Print and shaded views of the part. All mm, measured from the part's lowest x, y and z. A direction names the side the tool comes from. Round coordinates to 2 decimals unless told otherwise and drop trailing zeros. Loops run counter-clockwise (first coordinate to the right, second up) from the corner with the lowest first, then second, coordinate; pieces in that order, holes last. Notation, with made-up numbers: (25, 78) -> (58, 78) arc R26 ccw to (58, 96) -> close; hole circle Ø8 at (-14, 58.25). An arc over 180 degrees is marked (long way). Answer as CSV lines item,"result".
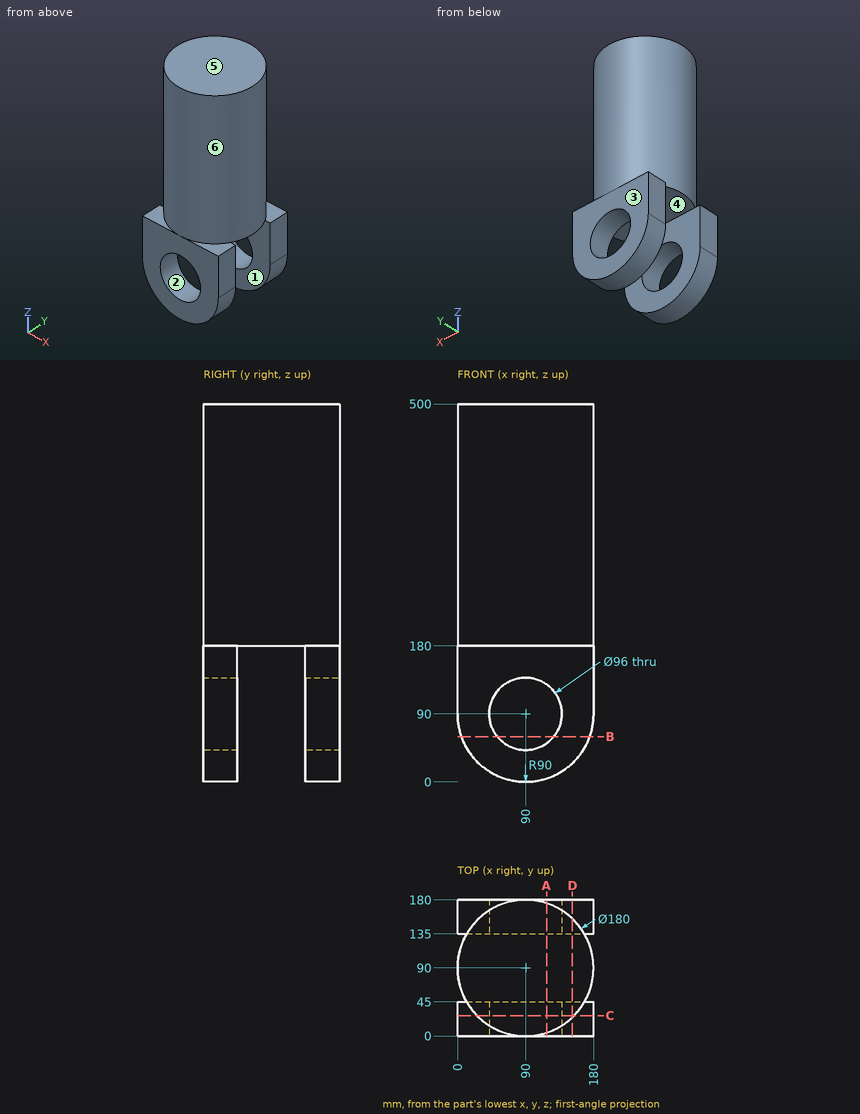
Q1. Drop flat-ended pins along their axis: pin 1 Ø8 at (x, y) = (55.5, 110.5) entering from -Z; pin 2 Ø12 at (x, z) = (27, 105.5) entering from -Y; pin 3 Ø1.5 at (x, z) = (84, 189.5) entering from +Y; pin 4 Ø1 at (x, z) = (69, 349.5) entering from +Y. Give the stop position or say it passes through.
Results:
pin 1,"z = 180"
pin 2,"y = 0"
pin 3,"y = 179.85"
pin 4,"y = 177.63"
Q2. Slice it at A-A, the plane x = 118. Give the cut face in (y, z), and give its area (3 significant figures).
Results:
outline,"(0, 4.47) -> (45, 4.47) -> (45, 51.01) -> (0, 51.01) -> close; (0, 128.99) -> (45, 128.99) -> (45, 180) -> (135, 180) -> (135, 128.99) -> (180, 128.99) -> (180, 180) -> (175.53, 180) -> (175.53, 500) -> (4.47, 500) -> (4.47, 180) -> (0, 180) -> close; (135, 4.47) -> (180, 4.47) -> (180, 51.01) -> (135, 51.01) -> close"
area,"63,500 mm2"
Q3. Slice it at C-C, the plane y = 27. Give the cut face in (x, z), and give its area (3 significant figures).
Results:
outline,"(0, 90) arc R90 ccw to (180, 90) -> (180, 180) -> (154.27, 180) -> (154.27, 500) -> (25.73, 500) -> (25.73, 180) -> (0, 180) -> close; hole circle Ø96 at (90, 90)"
area,"62,800 mm2"
Q4. Probe L1, parallel to Z at x = 90, y = 145; L2, parallel to X at y = 9, z = 90; L3, parallel to Y at x = 137.5, z = 161. List the from-to ranges inside material, lowest first. Write a range as [from, to].
Results:
L1,"[0, 42], [138, 500]"
L2,"[0, 42], [138, 180]"
L3,"[0, 45], [135, 180]"
Q5. Two-plate mould, pull along Y, no slides. Class the marked faces 1, 2 and 3: pulls with the +Y half, pulls with the -Y half, needs draft (parallel to the pull), parting line crosses it, or undercut.
Results:
face 1,"undercut"
face 2,"needs draft"
face 3,"pulls with the +Y half"
Q6. Slice it at B-B, the plane z = 60. Give the cut face in (x, y), and give its area (3 significant figures).
Results:
outline,"(5.15, 0) -> (52.53, 0) -> (52.53, 45) -> (5.15, 45) -> close; (5.15, 135) -> (52.53, 135) -> (52.53, 180) -> (5.15, 180) -> close; (127.47, 0) -> (174.85, 0) -> (174.85, 45) -> (127.47, 45) -> close; (127.47, 135) -> (174.85, 135) -> (174.85, 180) -> (127.47, 180) -> close"
area,"8,530 mm2"
Q7. Slice it at D-D, the plane x = 152. Give the cut face in (y, z).
Results:
outline,"(0, 24.76) -> (45, 24.76) -> (45, 180) -> (135, 180) -> (135, 24.76) -> (180, 24.76) -> (180, 180) -> (155.24, 180) -> (155.24, 500) -> (24.76, 500) -> (24.76, 180) -> (0, 180) -> close"
Q8. Tool access for the marked faces 4, 5 and 6: list every direction of +Z, -Z, +X, -X, +Y, -Y with a clear straight run to the whole face (end or side of a thin tool).
Results:
face 4,"-Z, +X, -X"
face 5,"+Z, +X, -X, +Y, -Y"
face 6,"+Z"
